Read the model definition and answer for the solid it produces. Units are mm, in the model's axes. A direction names the side the tool comes from. Coordinates: 2 decimals unless noted, no trailing zeros. Write each loop counter-clockwise with the first axis right and the second up, starting at its lowest first coordinate (ties: lowest second). Pieces come first, ordered by that corner, then holes. Notation, with made-up numbers: (-16, 29.5) -> (-6, 29.5) arc R29 ccw to (-6, 66.5) -> close; hole circle Ø1 at (-26, -3.75). An arc over 180 degrees is marked (long way). Return JSON: item names as keys, results as strings.
Autodesk Inventor part; units mm, degrees
ref_plane "YZ Plane" through (0, 0, 0) normal (1, 0, 0) x (0, 1, 0)
ref_plane "XZ Plane" through (0, 0, 0) normal (0, 1, 0) x (-1, 0, 0)
ref_plane "XY Plane" through (0, 0, 0) normal (0, 0, 1) x (1, 0, 0)
ref_plane "작업 평면1" through (0, 0, 0) normal (0, 0, 1) x (1, 0, 0)
sketch "스케치1" plane through (0, 0, 0) normal (0, 0, 1) x (1, 0, 0)
  line L0 (14.6, 27) -> (14.6, -35)
  line L1 (14.6, -35) -> (24.6, -35)
  line L2 (24.6, -35) -> (24.6, 35)
  line L3 (24.6, 35) -> (-24.6, 35)
  line L4 (-24.6, 35) -> (-24.6, -35)
  line L5 (-24.6, -35) -> (-14.6, -35)
  line L6 (-14.6, -35) -> (-14.6, 27)
  line L7 (-14.6, 27) -> (14.6, 27)
  circle A0 centre (-14.6, 30) radius 1.35
  circle A1 centre (14.6, 30) radius 1.35
  circle A2 centre (-17.3, -31) radius 1.35
  circle A3 centre (-17.3, 13) radius 1.35
  circle A4 centre (-17.3, -9) radius 1.35
  circle A5 centre (17.3, -9) radius 1.35
  circle A6 centre (17.3, 13) radius 1.35
  circle A7 centre (17.3, -31) radius 1.35
  line L8 (-24.6, 26) -> (24.6, 26)
  line L9 (24.6, 26) -> (24.6, 64)
  line L10 (-24.6, 64) -> (-24.6, 26)
  line L11 (22.1, 41.9) -> (16, 41.9)
  line L12 (16, 41.9) -> (16, 54)
  line L13 (16, 54) -> (22.1, 54)
  line L14 (22.1, 54) -> (22.1, 41.9)
  line L15 (8.1, 55) -> (-4, 55)
  line L16 (-4, 55) -> (-4, 61.1)
  line L17 (-4, 61.1) -> (8.1, 61.1)
  line L18 (8.1, 61.1) -> (8.1, 55)
  line L19 (-4, 64) -> (24.6, 64)
  line L20 (-24.6, 64) -> (-4, 64)
  point P0 (0, 0)
  dimension "d1" = 6.1
  dimension "d2" = 12.1
  dimension "d11" = 6.1
extrude "돌출2" add sketch "스케치1" along normal blind 6 contours L7 L6 L8 L4 L3 L2 L0 | L0 L8 L6 L7 | L3 L10 L20 L19 L9
sketch "스케치2" plane through (0, 0, 0) normal (0, 0, -1) x (-1, 0, 0)
  line L0 (-8.1, 61.1) -> (-8.1, 55)
  circle A0 centre (-13.1, 58) radius 1.35
  circle A1 centre (13.1, 58) radius 1.35
  point P0 (0, 0)
  dimension "d14" = 2.7
  dimension "d15" = 2.7
extrude "돌출3" cut sketch "스케치2" against normal through all
sketch "스케치3" plane through (0, 0, 6) normal (0, 0, 1) x (1, 0, 0)
  line L0 (8.1, 55) -> (-4, 55)
  line L1 (8.1, 61.1) -> (8.1, 55)
  line L2 (-4, 61.1) -> (8.1, 61.1)
  line L3 (-4, 55) -> (-4, 61.1)
  line L4 (16, 54) -> (22.1, 54)
  line L5 (22.1, 41.9) -> (16, 41.9)
  line L6 (22.1, 54) -> (22.1, 41.9)
  line L7 (16, 41.9) -> (16, 54)
  circle A0 centre (-4, 61.1) radius 1
  circle A1 centre (8.1, 61.1) radius 1
  circle A2 centre (8.1, 55) radius 1
  circle A3 centre (-4, 55) radius 1
  circle A4 centre (16, 54) radius 1
  circle A5 centre (22.1, 54) radius 1
  circle A6 centre (22.1, 41.9) radius 1
  circle A7 centre (16, 41.9) radius 1
  point P0 (0, 0)
  point P1 (22.1, 53)
  point P2 (21.1, 54)
  dimension "d18" = 2
  dimension "d19" = 2
  dimension "d20" = 2
  dimension "d21" = 2
  dimension "d22" = 2
  dimension "d23" = 2
  dimension "d24" = 2
  dimension "d25" = 2
extrude "돌출4" cut sketch "스케치3" against normal blind 10 contours A3 L3 L0 | L0 L3 A3 | A2 L1 L0 | L0 L1 A2 | A0 L2 L3 | L3 L2 A0 | A1 L2 L1 | L1 L2 A1 | L7 A4 L4 | L4 A4 L7 | A5 L6 L4 | A7 L5 L7 | L7 L5 A7 | A6 L5 L6 | L6 L5 A6 picked at (21.7924, 54.586)
properties part number "battery sideplate" material "PMMA 플라스틱"
1. The part is cut by section B-B (z = 3.65). Determine the outline of the cut face in (x, y), then the cut area to 3 significant figures.
Taken from the geometry:
{"outline": "(-24.6, 26) -> (24.6, 26) -> (24.6, 64) -> (-24.6, 64) -> close; hole circle Ø2.7 at (-14.6, 30); hole circle Ø2.7 at (-13.1, 58); hole (-4, 56) arc R1 ccw (long way) to (-3, 55) -> (7.1, 55) arc R1 ccw (long way) to (8.1, 56) -> (8.1, 60.1) arc R1 ccw (long way) to (7.1, 61.1) -> (-3, 61.1) arc R1 ccw (long way) to (-4, 60.1) -> close; hole circle Ø2.7 at (13.1, 58); hole circle Ø2.7 at (14.6, 30); hole (16, 42.9) arc R1 ccw (long way) to (17, 41.9) -> (21.1, 41.9) arc R1 ccw (long way) to (22.1, 42.9) -> (22.1, 53) arc R1 ccw (long way) to (21.1, 54) -> (17, 54) arc R1 ccw (long way) to (16, 53) -> close", "area": "1,680 mm2"}
2. For a pull along Y with two mould halves and no side action, classify faces 1 (the face through (24.6, 45, 3)), 2 (the face through (-4, 58, 3)), 3 (the face through (0, 64, 3)) as +Y half, -Y half, draft (parallel to the pull), parting line (faces both ways), or undercut.
Taken from the geometry:
{"face 1": "draft", "face 2": "undercut", "face 3": "+Y half"}
3. The part is cut by section D-D (x = 6). Determine the outline of the cut face in (y, z).
Taken from the geometry:
{"outline": "(26, 0) -> (55, 0) -> (55, 6) -> (26, 6) -> close; (61.1, 0) -> (64, 0) -> (64, 6) -> (61.1, 6) -> close"}
4. A flat-ended cylindrical pin translates along its axis: pin 1 Ø1.6 at (x, y) = (-4, 61.1) entering from -Z. Find the tip coordinate at first contact, or state that the pin passes through.
Taken from the geometry:
{"pin 1": "passes through"}
5. A tool of negligible diameter and unlimited length cuts with its end or side. For faces 4 (the face through (-24.6, 45, 3)), 5 (the face through (16, 48, 3)), from which of +Z, -Z, +X, -X, +Y, -Y can it reach the whole face along a straight path? Write none if from no direction.
Taken from the geometry:
{"face 4": "+Z, -Z, -X, +Y, -Y", "face 5": "+Z, -Z"}
6. Consider L1, parallel to X at y = 61, z = 2.7; L2, parallel to X at y = 52.5, z = 3; L3, parallel to Y at x = -13.1, z = 2.65. Determine where each line is inside the solid, lowest interval first.
Taken from the geometry:
{"L1": "x = -24.6 to -4.99, 9.09 to 24.6", "L2": "x = -24.6 to 16, 22.1 to 24.6", "L3": "y = 26 to 56.65, 59.35 to 64"}
7. The part is cut by section A-A (y = 48.5). Determine the outline of the cut face in (x, z).
Taken from the geometry:
{"outline": "(-24.6, 0) -> (16, 0) -> (16, 6) -> (-24.6, 6) -> close; (22.1, 0) -> (24.6, 0) -> (24.6, 6) -> (22.1, 6) -> close"}
8. The part is cut by section C-C (y = 58). Determine the outline of the cut face in (x, z), then the cut area to 3 significant figures.
Taken from the geometry:
{"outline": "(-24.6, 0) -> (-14.45, 0) -> (-14.45, 6) -> (-24.6, 6) -> close; (-11.75, 0) -> (-4, 0) -> (-4, 6) -> (-11.75, 6) -> close; (8.1, 0) -> (11.75, 0) -> (11.75, 6) -> (8.1, 6) -> close; (14.45, 0) -> (24.6, 0) -> (24.6, 6) -> (14.45, 6) -> close", "area": "190 mm2"}
